Verification items for the finished model (mm, model axes). A direction names the side the tool comes from. Coordinates: 2 decimals unless noted, no trailing zeros. Order: outer loops, then holes, each group sorted by start corner. A loop starts at its lowest first (then second) coordinate and runs counter-clockwise, first axis right, second up.
Q1. Cross-section at B-B, the plane x = -193.5. Record the boundary of the cut face in (y, z), and give its area (3 significant figures).
Q2. Thickness scan on line 1 (Z direction, x = -167, y = 47); line 2 (X direction, y = 42, z = -264); line 3 (Z direction, x = -176.5, y = 51). Record the ranges inside material, lowest first.
Q3. Cross-section at A-A, the plane z = -217.5. Record the boundary of the cut face in (x, y).
Q4. Draft check along Z on faces 1 (the flat face through (-149.75, 28, -214)), 2 (the flat face through (-187, 25, 0)), 3 (the flat face through (-145, 0, -212)), 4 (the flat face through (-249.75, 28, -216)). Enter one of: pulls with the +Z half, pulls with the -Z half, needs draft (parallel to the pull), parting line crosses it, or undercut.
Q5. Depth check by flat-ended pin: P1, Ø10, axis at x = -148.5, y = 18, coming from the +Z side; P2, Ø2.5, axis at y = 53.5, z = -265, coming from the -X side; P3, Ø4, axis at x = -169, y = 54, coming from the +Z side; P4, Ø2.5, axis at y = 53, z = -242, coming from the +X side. Enter the tip coordinate at first touch or a pass-through.
Q6. Cross-section at C-C, the plane y = 43. Record the boundary of the cut face in (x, z).
Q7. Set-up check for faces 5 (the flat face through (-199, 28, -290)), 6 (the flat face through (0, 25, -218)): record each of +Z, -Z, +X, -X, +Y, -Y from which the full face is reachable in a straight line by a thin tool's end or side.
Q8. Cross-section at D-D, the plane z = -76. Record the boundary of the cut face in (x, y), and give its area (3 significant figures).
Autodesk Inventor part; units mm, degrees
ref_plane "YZ Plane" through (0, 0, 0) normal (1, 0, 0) x (0, 1, 0)
ref_plane "XZ Plane" through (0, 0, 0) normal (0, 1, 0) x (-1, 0, 0)
ref_plane "XY Plane" through (0, 0, 0) normal (0, 0, 1) x (1, 0, 0)
sketch "Sketch1" plane through (0, 0, 0) normal (0, 1, 0) x (-1, 0, 0)
  line L0 (0, 0) -> (380, 0)
  line L1 (380, 0) -> (380, -430)
  line L2 (380, -430) -> (0, -430)
  line L3 (0, -430) -> (0, 0)
  line L4 (249.75, -140) -> (149.75, -140)
  line L5 (149.75, -140) -> (149.75, -290)
  line L6 (149.75, -290) -> (249.75, -290)
  line L7 (249.75, -290) -> (249.75, -140)
  dimension "d0" = 380
  dimension "d1" = 430
  dimension "d2" = 100
  dimension "d3" = 150
  dimension "d4" = 140
  dimension "d5" = 149.75
extrude "Extrusion1" add sketch "Sketch1" along normal blind 50.8
sketch "Sketch5" plane through (0, 50.8, 0) normal (0, 1, 0) x (1, 0, 0)
  line L0 (-349.5, 38) -> (-50, 38)
  line L1 (-50, 38) -> (-50, 392)
  line L2 (-50, 392) -> (-349.5, 392)
  line L3 (-349.5, 392) -> (-349.5, 38)
  line L4 (-380, 0) -> (0, 0)
  line L5 (-380, 430) -> (-380, 0)
  line L6 (-249.75, 140) -> (-149.75, 140)
  line L7 (-149.75, 290) -> (-249.75, 290)
  line L8 (-249.75, 140) -> (-149.75, 140)
  line L9 (-149.75, 140) -> (-149.75, 290)
  line L10 (-149.75, 290) -> (-249.75, 290)
  line L11 (-249.75, 290) -> (-249.75, 140)
  dimension "d14" = 299.5
  dimension "d15" = 354
  dimension "d16" = 38
  dimension "d17" = 30.5
extrude "Extrusion2" add sketch "Sketch5" along normal blind 5
properties part number "TapaFrontal"
Check values:
1. outline: (0, -430) - (50.8, -430) - (50.8, -392) - (55.8, -392) - (55.8, -290) - (0, -290) - close; (0, -140) - (55.8, -140) - (55.8, -38) - (50.8, -38) - (50.8, 0) - (0, 0) - close
1. area: 15,200 mm2
2. line 1: z = -430 to -290, -140 to 0
2. line 2: x = -380 to -249.75, -149.75 to 0
2. line 3: z = -392 to -290, -140 to -38
3. outline: (-380, 0) - (-249.75, 0) - (-249.75, 55.8) - (-349.5, 55.8) - (-349.5, 50.8) - (-380, 50.8) - close; (-149.75, 0) - (0, 0) - (0, 50.8) - (-50, 50.8) - (-50, 55.8) - (-149.75, 55.8) - close
4. face 1: undercut
4. face 2: pulls with the +Z half
4. face 3: needs draft
4. face 4: undercut
5. P1: stops at z = 0
5. P2: stops at x = -349.5
5. P3: stops at z = -38
5. P4: stops at x = -50
6. outline: (-380, -430) - (0, -430) - (0, 0) - (-380, 0) - close; hole (-249.75, -290) - (-149.75, -290) - (-149.75, -140) - (-249.75, -140) - close
7. face 5: +Y, -Y
7. face 6: +Z, -Z, +X, +Y, -Y
8. outline: (-380, 0) - (0, 0) - (0, 50.8) - (-50, 50.8) - (-50, 55.8) - (-349.5, 55.8) - (-349.5, 50.8) - (-380, 50.8) - close
8. area: 20,800 mm2
